```python
from build123d import *

# Parameters (mm, degrees)
BOSS_EXTRUDE1_DEPTH = 270
CUT_EXTRUDE1_REACH  = 509.382
SKETCH2_R           = 180


with BuildPart() as part:
    # Sketch1 → Boss-Extrude1 (new, symmetric)
    with BuildSketch(Plane.XY):
        Polygon((-414.487497153, -33.008195855), (412.751015377, 112.856273385), (413.619256265, 107.93223462), (-413.619256265, -37.93223462), align=None)
    extrude(amount=BOSS_EXTRUDE1_DEPTH, both=True)

    # Cut-Extrude1: up to this face of the body (flat: up to its plane)
    cut_extrude1_end = Plane(part.part.faces().sort_by_distance((-0.868240888, 39.924038765, 0))[0])
    # Sketch2 → Cut-Extrude1 (cut, up to the picked face)
    with BuildSketch(Plane(origin=(0, 0, 0), x_dir=(1, 0, 0), z_dir=(0, 1, 0)), mode=Mode.PRIVATE) as cut_extrude1_sk1:
        with Locations(Location((0, 0, 0), (0, 0, 180))):
            Circle(SKETCH2_R)
    cut_extrude1_tool1 = split(extrude(cut_extrude1_sk1.sketch, amount=CUT_EXTRUDE1_REACH, mode=Mode.PRIVATE), bisect_by=cut_extrude1_end, keep=Keep.BOTH, mode=Mode.PRIVATE)
    add(cut_extrude1_tool1.solids().sort_by(Axis((0, 0, 0), (0, 1, 0)))[0], mode=Mode.SUBTRACT)


solid = part.part
```
The model under review builds one solid part; all positions refer to its coordinate system, in mm. Round coordinates to 2 decimals unless told otherwise and drop trailing zeros. Order: outer loops, then holes, each group sorted by start corner. A loop starts at its lowest first (then second) coordinate and runs counter-clockwise, first axis right, second up. Notation, with made-up numbers: (3, 75.5) -> (21, 75.5) arc R5 cw to (21, 83.5) -> close; hole circle Ø5 at (-21.75, 65). An arc over 180 degrees is marked (long way). One line per item, written item: value. Start each with the question number.
Q1. Wall thickness on line 1 (Z direction, x = 0, y = 39); line 2 (Y direction, x = 188.5, z = 84); line 3 (Y direction, x = 193.5, z = -176): over which ranges is each line inside the solid? List them lowest first.
Q2. Clearance check with flat-ended pins moving along their axes: pin 1 Ø1 at (y, z) = (63.5, 78.5) entering from -X; pin 2 Ø8 at (x, z) = (-238, -64.5) entering from +Y; pin 3 Ø4 at (x, z) = (291.5, -40.5) entering from +Y. State where each tip first meets the part, or that it passes through.
Q3. Mouldability with a two-part tool opening along Z and no side actions: class faces 1 (the face through (1, 38, -270)), 2 (the face through (-87.705, 22.257, -157.187)), 3 (the face through (1, 38, 270)), 4 (the face through (5.79, 36.02, 183.78)) as released by +Z, released by -Z, zero draft, split by the parting line, or undercut.
Q4. Take a section at C-C (z = -233.5). Write out the cut boundary in (x, y), and give its area (3 significant figures).
Q5. Take a section at D-D (y = -24). Write out the cut boundary in (x, z).
Q6. Take a section at B-B (x = -42). Write out the cut boundary in (y, z).
Q7. Take a section at A-A (z = 0). Write out the cut boundary in (x, y).
Reported:
1. line 1: z = -270 to -180, 180 to 270
1. line 2: y = 68.24 to 73.31
1. line 3: y = 69.12 to 74.2
2. pin 1: stops at x = 161.74
2. pin 2: stops at y = -1.18
2. pin 3: stops at y = 91.83
3. face 1: released by -Z
3. face 2: undercut
3. face 3: released by +Z
3. face 4: zero draft
4. outline: (-414.49, -33.01) -> (-413.62, -37.93) -> (413.62, 107.93) -> (412.75, 112.86) -> close
4. area: 4,200 mm2
5. outline: (-363.4, -270) -> (-334.61, -270) -> (-334.61, 270) -> (-363.4, 270) -> close
6. outline: (27.59, -270) -> (32.67, -270) -> (32.67, -175.03) -> (27.59, -175.03) -> close; (27.59, 175.03) -> (32.67, 175.03) -> (32.67, 270) -> (27.59, 270) -> close
7. outline: (-414.49, -33.01) -> (-413.62, -37.93) -> (-180, 3.26) -> (-180, 8.34) -> close; (180, 66.74) -> (413.62, 107.93) -> (412.75, 112.86) -> (180, 71.82) -> close
